Read the model definition and answer for the solid it produces. Units are mm, in the model's axes. Face numbers are marked on the shaded views. Coordinates: 2 decimals unless noted, no trailing zeros. Loops run counter-clockwise (first coordinate to the right, second up) from the corner with the lowest first, then second, coordinate; pieces in that order, holes last. Notation, with made-up numbers: (-34.75, 79.5) -> (-9.75, 79.5) arc R12 cw to (-9.75, 83.5) -> close; hole circle Ø5 at (35.25, 43.5). An arc over 180 degrees is marked (long way). Answer as a JSON object with one key per item and string values. Group by question number.
1) Section C-C, the plane z = -4.5 is taken. Give the vertices of the cut face in (x, y) (3 decimals).
2) Section B-B, the plane y = 4.25 is taken. Give the vertices of the cut face in (x, z).
3) Section D-D, the plane z = -23.5 is taken. Give the vertices of the cut face in (x, y) (3 decimals).
4) Consider probe 1 along X at (y, z) = (2.5, -4.5); probe 2 along Z at (x, y) = (38.5, 2.75); probe 3 along X at (y, z) = (3, -23.5). Determine where each line is inside the solid, lowest interval first. Write a range as [from, to].
5) Determine the mould class of the marked faces 1, 2 and 3 for opening direction Z: released by +Z, released by -Z, zero draft, split by the parting line, or undercut.
6) Section A-A, the plane x = 23.5 is taken. Give the vertices of the cut face in (y, z) (3 decimals), plus the area to 3 significant figures.
7) A flat-ended cylindrical pin translates along its axis: P1, Ø4, axis at x = 38.5, z = -4.5, coming from the +Y side. Find the tip coordinate at first contact, or state that the pin passes through.
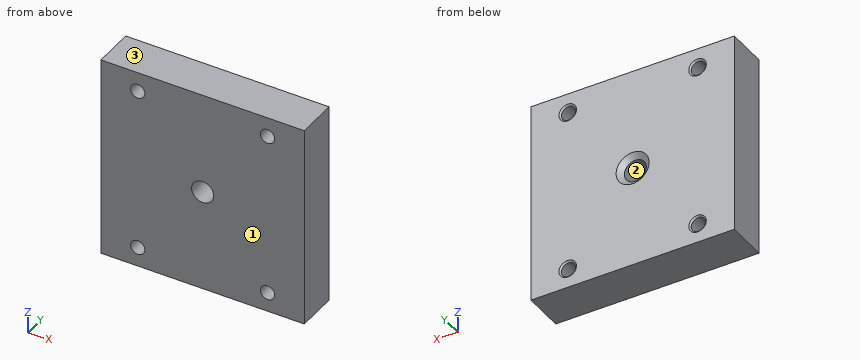
from build123d import *

# Parameters (mm, degrees)
SKETCH1_W                         = 47
SKETCH1_H                         = 47
BOSS_EXTRUDE1_DEPTH               = 9.525
M4X0_7_TAPPED_HOLE1_D             = 3.3
M4X0_7_TAPPED_HOLE1_CSINK_D       = 4.05
M4X0_7_TAPPED_HOLE1_CSINK_ANGLE   = 100
F_1_4_20_TAPPED_HOLE1_D           = 5.1054
F_1_4_20_TAPPED_HOLE1_CSINK_D     = 7.62
F_1_4_20_TAPPED_HOLE1_CSINK_ANGLE = 100


with BuildPart() as part:
    # Sketch1 → Boss-Extrude1 (new body)
    with BuildSketch(Plane(origin=(0, 0, 0), x_dir=(1, 0, 0), z_dir=(0, 1, 0))):
        with Locations((23.5, 23.5)):
            Rectangle(SKETCH1_W, SKETCH1_H)
    extrude(amount=BOSS_EXTRUDE1_DEPTH)

    # M4x0.7 Tapped Hole1 (through all)
    with Locations(Plane(origin=(0, 9.525, 0), x_dir=(1, 0, 0), z_dir=(0, 1, 0))):
        with Locations((38.5, 42.5), (8.5, 42.5), (8.5, 4.5), (38.5, 4.5)):
            CounterSinkHole(M4X0_7_TAPPED_HOLE1_D / 2, M4X0_7_TAPPED_HOLE1_CSINK_D / 2, counter_sink_angle=M4X0_7_TAPPED_HOLE1_CSINK_ANGLE)

    # 1/4-20 Tapped Hole1 (through all)
    with Locations(Plane(origin=(0, 9.525, 0), x_dir=(1, 0, 0), z_dir=(0, 1, 0))):
        with Locations((23.5, 23.5)):
            CounterSinkHole(F_1_4_20_TAPPED_HOLE1_D / 2, F_1_4_20_TAPPED_HOLE1_CSINK_D / 2, counter_sink_angle=F_1_4_20_TAPPED_HOLE1_CSINK_ANGLE)


solid = part.part
Determined:
{
 "1": {"outline": "(0, 0) -> (6.85, 0) -> (6.85, 9.21) -> (6.475, 9.525) -> (0, 9.525) -> close; (10.15, 0) -> (36.85, 0) -> (36.85, 9.21) -> (36.475, 9.525) -> (10.525, 9.525) -> (10.15, 9.21) -> close; (40.15, 0) -> (47, 0) -> (47, 9.525) -> (40.525, 9.525) -> (40.15, 9.21) -> close"},
 "2": {"outline": "(0, -47) -> (47, -47) -> (47, 0) -> (0, 0) -> close; hole circle Ø3.3 at (8.5, -42.5); hole circle Ø3.3 at (8.5, -4.5); hole circle Ø5.11 at (23.5, -23.5); hole circle Ø3.3 at (38.5, -42.5); hole circle Ø3.3 at (38.5, -4.5)"},
 "3": {"outline": "(0, 0) -> (20.947, 0) -> (20.947, 8.47) -> (19.69, 9.525) -> (0, 9.525) -> close; (26.053, 0) -> (47, 0) -> (47, 9.525) -> (27.31, 9.525) -> (26.053, 8.47) -> close"},
 "4": {"probe 1": "[0, 6.85], [10.15, 36.85], [40.15, 47]", "probe 2": "[-47, -44.15], [-40.85, -6.15], [-2.85, 0]", "probe 3": "[0, 20.95], [26.05, 47]"},
 "5": {"face 1": "zero draft", "face 2": "undercut", "face 3": "released by +Z"},
 "6": {"outline": "(0, -47) -> (9.525, -47) -> (9.525, -27.31) -> (8.47, -26.053) -> (0, -26.053) -> close; (0, -20.947) -> (8.47, -20.947) -> (9.525, -19.69) -> (9.525, 0) -> (0, 0) -> close", "area": "398 mm²"},
 "7": {"P1": "y = 9.5"}
}
